Print and shaded views of the part. All mm, measured from the part's lowest x, y and z. Give positions to 0.01 mm unless a question says otherwise; leave off trailing zeros. Loops run counter-clockwise (first coordinate to the right, second up) from the corner with the lowest first, then second, coordinate; pieces in that order, holes last.
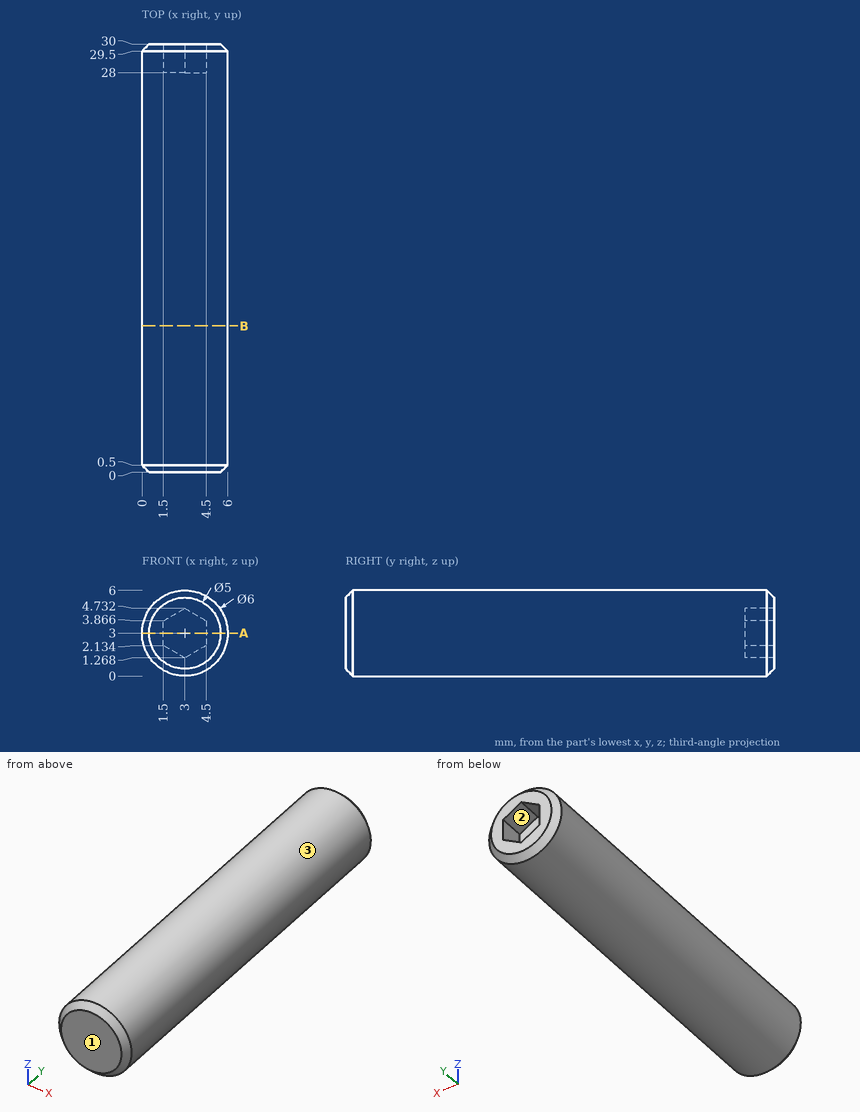
1. Saw through at A-A, the plane z = 3. List the corners of the cut face in (x, y).
Responses:
outline: (0, 0.5) - (0.5, 0) - (5.5, 0) - (6, 0.5) - (6, 29.5) - (5.5, 30) - (4.5, 30) - (4.5, 28) - (1.5, 28) - (1.5, 30) - (0.5, 30) - (0, 29.5) - close
2. Pull direction X, two halves, no side cores. Call the marked faces 1, 2 and 3: released by +X, released by -X, zero draft, split by the parting line, or undercut.
Responses:
face 1: zero draft
face 2: undercut
face 3: split by the parting line
3. Probe line 1 along Z through (x, y) = (3.1, 1); line 2 along Y through (x, z) = (4, 2.6); line 3 along Z through (x, y) = (3.95, 28.75). List the from-to ranges inside material, lowest first.
Responses:
line 1: z = 0 to 6
line 2: y = 0 to 28
line 3: z = 0.15 to 1.82, 4.18 to 5.85
4. Saw through at B-B, the plane y = 10.25. List the corners of the cut face in (x, z).
Responses:
outline: circle Ø6 at (3, 3)
5. Drop flat-ended pins along their axis: pin 1 (1 mm diameter, centred on y = 19.5, z = 1.5, fed in from +X); pin 2 (1.5 mm diameter, centred on y = 10.5, z = 1.5, fed in from -X); pin 3 (1.5 mm diameter, centred on y = 17.5, z = 4.5, fed in from +X). Give the stop position or say it passes through.
Responses:
pin 1: stops at x = 5.83
pin 2: stops at x = 0.1
pin 3: stops at x = 5.9
